from build123d import *

# Parameters (mm, degrees)
SKETCH_1_R           = 2.250000000000002
SKETCH_1_R_2         = 2.2500000000000027
EXTRUDE_1_DEPTH      = 4
EXTRUDE_2_DEPTH      = 58
EXTRUDE_3_REACH      = 110.805
EXTRUDE_3_END_RADIUS = 44.19999999999999
CUT_EXTRUDE_1_REACH  = 89.17
SKETCH_4_R           = 3.0000000000000013
FILLET_1_R           = 2
CHAMFER_1_SIZE       = 2
EXTRUDE_4_DEPTH      = 58
EXTRUDE_5_DEPTH      = 6.412205295
SKETCH_8_R           = 1.5000000000000042
SKETCH_8_R_2         = 1.5000000000000009
SKETCH_8_R_3         = 1.500000000000004
SKETCH_8_R_4         = 1.500000000000017
SKETCH_8_R_5         = 1.5000000000000173
CUT_EXTRUDE_2_DEPTH  = 5
CHAMFER_2_SIZE       = 0.5
CHAMFER_3_SIZE       = 3


with BuildPart() as part:
    # Эскиз1 → Бобышка-Вытянуть1 (new body)
    with BuildSketch(Plane(origin=(0, 0, 0), x_dir=(1, 0, 0), z_dir=(0, 1, 0))):
        with BuildLine():
            Line((-42.93077537059159, -10.516107934012744), (-39.47597367549217, -16.5))
            Line((-39.47597367549216, -16.5), (-34.49999999999999, -16.5))
            Line((-34.49999999999999, -16.5), (-34.49999999999999, -3.5000000000000013))
            Line((-34.49999999999999, -3.5000000000000013), (-34.49999999999999, 3.5000000000000013))
            Line((-34.49999999999999, 3.5000000000000018), (-34.49999999999999, 17.5))
            Line((-34.49999999999999, 17.5), (-25.274990747593094, 17.499999999999996))
            Line((-25.274990747593094, 17.499999999999996), (-16, 26.77499074759315))
            Line((-16, 26.77499074759315), (16, 26.77499074759315))
            Line((16, 26.77499074759315), (25.274990747593094, 17.499999999999996))
            Line((25.274990747593094, 17.499999999999996), (34.50000000000001, 17.5))
            Line((34.50000000000001, 17.5), (34.50000000000001, 3.5000000000000013))
            Line((34.50000000000001, 3.5000000000000013), (34.5, -3.5000000000000013))
            Line((34.5, -3.5000000000000018), (34.5, -16.5))
            Line((34.5, -16.5), (39.475973675492156, -16.5))
            Line((39.475973675492156, -16.5), (42.9307753705916, -10.516107934012684))
            ThreePointArc((42.93077537059159, -10.516107934012682), (44.199999999999974, 1.599e-14), (42.93077537059159, 10.516107934012718))
            Line((42.93077537059159, 10.516107934012716), (30.572604305089854, 31.92108810808932))
            ThreePointArc((30.57260430508986, 31.92108810808933), (22.099999999999994, 38.27832284727222), (12.358171065501741, 42.43719604210199))
            Line((12.358171065501741, 42.437196042101974), (-12.358171065501741, 42.437196042101974))
            ThreePointArc((-12.358171065501743, 42.43719604210198), (-22.099999999999994, 38.278322847272186), (-30.572604305089868, 31.921088108089307))
            Line((-30.572604305089865, 31.9210881080893), (-42.930775370591604, 10.5161079340127))
            ThreePointArc((-42.930775370591604, 10.516107934012702), (-44.19999999999999, -1.954e-14), (-42.93077537059159, -10.516107934012746))
        make_face()
        with Locations(Location((-39, 0, 0), (0, 0, 270))):
            Circle(SKETCH_1_R, mode=Mode.SUBTRACT)
        with Locations(Location((39, 0, 0), (0, 0, 270))):
            Circle(SKETCH_1_R, mode=Mode.SUBTRACT)
        with Locations(Location((-19.50000000000016, 33.77499074759302, 0), (0, 0, 270))):
            Circle(SKETCH_1_R_2, mode=Mode.SUBTRACT)
        with BuildLine():
            Line((-8, 36.024990747593144), (8, 36.024990747593144))
            ThreePointArc((8, 36.024990747593144), (10.25, 33.774990747593144), (7.999999999999998, 31.524990747593144))
            Line((7.999999999999998, 31.524990747593144), (-7.999999999999998, 31.524990747593144))
            ThreePointArc((-7.999999999999998, 31.524990747593144), (-10.25, 33.774990747593144), (-8, 36.024990747593144))
        make_face(mode=Mode.SUBTRACT)
        with Locations(Location((19.499999999999925, 33.77499074759315, 0), (0, 0, 270))):
            Circle(SKETCH_1_R_2, mode=Mode.SUBTRACT)
    extrude(amount=EXTRUDE_1_DEPTH)

    # Эскиз2 → Бобышка-Вытянуть2 (add)
    with BuildSketch(Plane(origin=(0, 4, 0), x_dir=(1, 0, 0), z_dir=(0, 1, 0))):
        with BuildLine():
            ThreePointArc((-42.9307753705916, 10.516107934012743), (-43.16465657781108, 9.51064784962775), (-43.37499279538843, 8.50000000000001))
            Line((-43.37499279538844, 8.50000000000001), (-34.499999999999986, 8.500000000000005))
            Line((-34.499999999999986, 8.500000000000005), (-34.49999999999999, 16.5))
            Line((-34.49999999999999, 16.5), (-39.47597367549217, 16.5))
            Line((-39.47597367549217, 16.5), (-42.9307753705916, 10.516107934012743))
        make_face()
        with BuildLine():
            Line((-34.499999999999986, -8.500000000000005), (-43.37499279538844, -8.50000000000001))
            ThreePointArc((-43.37499279538843, -8.50000000000001), (-43.16465657781108, -9.51064784962775), (-42.9307753705916, -10.516107934012743))
            Line((-42.9307753705916, -10.516107934012743), (-39.47597367549217, -16.5))
            Line((-39.47597367549217, -16.5), (-34.49999999999999, -16.5))
            Line((-34.49999999999999, -16.5), (-34.499999999999986, -8.500000000000005))
        make_face()
        with BuildLine():
            Line((34.499999999999986, 8.500000000000005), (43.37499279538844, 8.50000000000001))
            ThreePointArc((43.37499279538845, 8.50000000000001), (43.16465657781109, 9.510647849627738), (42.930775370591604, 10.51610793401272))
            Line((42.930775370591604, 10.516107934012684), (39.475973675492156, 16.5))
            Line((39.475973675492156, 16.5), (34.5, 16.5))
            Line((34.5, 16.5), (34.499999999999986, 8.500000000000005))
        make_face()
        with BuildLine():
            ThreePointArc((42.93077537059162, -10.516107934012688), (43.164656577811115, -9.510647849627723), (43.37499279538845, -8.50000000000001))
            Line((43.37499279538844, -8.50000000000001), (34.499999999999986, -8.500000000000005))
            Line((34.499999999999986, -8.500000000000005), (34.5, -16.5))
            Line((34.5, -16.5), (39.475973675492156, -16.5))
            Line((39.475973675492156, -16.5), (42.930775370591604, -10.516107934012684))
        make_face()
    extrude(amount=EXTRUDE_2_DEPTH)

    # Бобышка-Вытянуть3: up to this cylinder (the profile starts inside it)
    extrude_3_end = Plane(origin=(0, 61.785199, 0), z_dir=(0, -1, 0)) * Cylinder(EXTRUDE_3_END_RADIUS, 311.01, mode=Mode.PRIVATE)
    # Эскиз3 → Бобышка-Вытянуть3 (add, up to the surface)
    with BuildSketch(Plane(origin=(-34.49999999999999, 0, 0), x_dir=(0, 0, -1), z_dir=(1, 0, 0)), mode=Mode.PRIVATE) as extrude_3_sk1:
        Polygon((-8.500000000000007, 62.00000000000001), (8.500000000000005, 62.00000000000001), (8.500000000000005, 48.87009446294909), (0, 59.00000000000001), (-8.500000000000005, 48.87009446294909), align=None)
    extrude_3_tool1 = extrude(extrude_3_sk1.sketch, amount=-EXTRUDE_3_REACH, mode=Mode.PRIVATE) & extrude_3_end
    extrude_3 = extrude_3_tool1.solids().sort_by_distance((-34.5, 61.785199, 0))[0]
    add(extrude_3)

    # Зеркальное отражение1: Бобышка-Вытянуть3 across plane
    add(extrude_3.mirror(Plane(origin=(0, 0, 0), x_dir=(0, 0, 1), z_dir=(1, 0, 0))))

    # Вырез-Вытянуть1: up to this face of the body (flat: up to its plane)
    cut_extrude_1_end = Plane(part.part.faces().sort_by_distance((44.00427315, 4, 0))[0])
    # Эскиз4 → Вырез-Вытянуть1 (cut, up to the picked face)
    with BuildSketch(Plane(origin=(0, 62.00000000000001, 0), x_dir=(1, 0, 0), z_dir=(0, 1, 0)), mode=Mode.PRIVATE) as cut_extrude_1_sk1:
        with Locations(Location((-39, 0, 0), (0, 0, 270))):
            Circle(SKETCH_4_R)
    cut_extrude_1_tool1 = split(extrude(cut_extrude_1_sk1.sketch, amount=-CUT_EXTRUDE_1_REACH, mode=Mode.PRIVATE), bisect_by=cut_extrude_1_end, keep=Keep.BOTH, mode=Mode.PRIVATE)
    # Эскиз4 → Вырез-Вытянуть1 (cut, up to the picked face)
    with BuildSketch(Plane(origin=(0, 62.00000000000001, 0), x_dir=(1, 0, 0), z_dir=(0, 1, 0)), mode=Mode.PRIVATE) as cut_extrude_1_sk2:
        with Locations(Location((39, 0, 0), (0, 0, 270))):
            Circle(SKETCH_4_R)
    cut_extrude_1_tool2 = split(extrude(cut_extrude_1_sk2.sketch, amount=-CUT_EXTRUDE_1_REACH, mode=Mode.PRIVATE), bisect_by=cut_extrude_1_end, keep=Keep.BOTH, mode=Mode.PRIVATE)
    add(cut_extrude_1_tool1.solids().sort_by(Axis((-39, 62, 0), (0, -1, 0)))[0], mode=Mode.SUBTRACT)
    add(cut_extrude_1_tool2.solids().sort_by(Axis((39, 62, 0), (0, -1, 0)))[0], mode=Mode.SUBTRACT)

    # Скругление1
    fillet_1_edges = [part.edges().sort_by_distance(p)[0] for p in [
        (35.249999999999986, 59.00000000000001, 0),
        (43.1, 59.00000000000001, 0),
        (-43.1, 59.00000000000001, 0),
        (-35.249999999999986, 59.00000000000001, 0),
    ]]
    fillet(fillet_1_edges, radius=FILLET_1_R)

    # Фаска1
    chamfer_1_edges = [part.edges().sort_by_distance(p)[0] for p in [
        (-19.50000000000016, 4, -36.02499074759302),
        (19.499999999999925, 4, -36.02499074759315),
        (39, 4, -2.250000000000002),
        (-39, 4, -2.250000000000002),
    ]]
    chamfer(chamfer_1_edges, length=CHAMFER_1_SIZE)

    # Эскиз6 → Бобышка-Вытянуть4 (add)
    with BuildSketch(Plane(origin=(0, 4, 0), x_dir=(1, 0, 0), z_dir=(0, 1, 0))):
        with BuildLine():
            Line((8, 36.024990747593144), (5.000000000000001, 36.024990747593144))
            Line((5.000000000000001, 36.024990747593144), (5, 42.437196042101974))
            Line((5, 42.437196042101974), (12.358171065501741, 42.437196042101974))
            ThreePointArc((12.358171065501741, 42.437196042101974), (14.696759256079767, 41.68507247647332), (16.989949980131733, 40.8041860557544))
            Line((16.989949980131733, 40.8041860557544), (15, 36.02499074759314))
            Line((15, 36.02499074759314), (8, 36.024990747593144))
        make_face()
        with BuildLine():
            Line((-12.358171065501741, 42.437196042101974), (-5, 42.437196042101974))
            Line((-5, 42.437196042101974), (-5.000000000000001, 36.024990747593144))
            Line((-5.000000000000001, 36.024990747593144), (-8, 36.024990747593144))
            Line((-8, 36.024990747593144), (-15, 36.02499074759314))
            Line((-15, 36.02499074759314), (-16.989949980131733, 40.8041860557544))
            ThreePointArc((-16.989949980131733, 40.8041860557544), (-14.696759256079767, 41.685072476473316), (-12.358171065501741, 42.437196042101974))
        make_face()
    extrude(amount=EXTRUDE_4_DEPTH)

    # Эскиз7 → Бобышка-Вытянуть5 (add)
    with BuildSketch(Plane.XY.offset(-36.024990747593144)):
        Polygon((-5.000000000000001, 62.00000000000001), (-5, 53.04123203702888), (0, 59.00000000000001), (5.000000000000003, 53.04123203702888), (5.000000000000001, 62.00000000000001), align=None)
    extrude(amount=-EXTRUDE_5_DEPTH)

    # Эскиз8 → Вырез-Вытянуть2 (cut)
    with BuildSketch(Plane(origin=(0, 62.00000000000001, 0), x_dir=(1, 0, 0), z_dir=(0, 1, 0))):
        with Locations(Location((38.99999999999992, 8, 0), (0, 0, 270))):
            Circle(SKETCH_8_R)
        with Locations(Location((8, 39.23109339484765, 0), (0, 0, 270))):
            Circle(SKETCH_8_R_2)
        with Locations(Location((38.99999999999992, -8, 0), (0, 0, 90))):
            Circle(SKETCH_8_R_3)
        with Locations(Location((-8, 39.23109339484765, 0), (0, 0, 90))):
            Circle(SKETCH_8_R)
        with Locations(Location((-38.999999999999865, -8.000000000000222, 0), (0, 0, 270))):
            Circle(SKETCH_8_R_4)
        with Locations(Location((-38.99999999999998, 7.999999999999556, 0), (0, 0, 90))):
            Circle(SKETCH_8_R_5)
    extrude(amount=-CUT_EXTRUDE_2_DEPTH, mode=Mode.SUBTRACT)

    # Фаска2
    chamfer_2_edges = [part.edges().sort_by_distance(p)[0] for p in [
        (8, 62.00000000000001, -40.73109339484765),
        (40.22474487139151, 62.00000000000001, 7.133974596215554),
        (-8, 62.00000000000001, -37.73109339484764),
        (-39.8660254037844, 62.00000000000001, 9.224744871391763),
        (-38.13397459621573, 62.00000000000001, -9.224744871391302),
        (37.775255128608336, 62.00000000000001, -7.133974596215554),
    ]]
    chamfer(chamfer_2_edges, length=CHAMFER_2_SIZE)

    # Фаска3
    chamfer_3_edges = [part.edges().sort_by_distance(p)[0] for p in [
        (-38.93749639769421, 4, 8.500000000000007),
        (38.93749639769421, 4, -8.500000000000007),
        (38.93749639769421, 4, 8.500000000000009),
        (5, 4, -39.23109339484756),
        (-5, 4, -39.23109339484756),
        (-38.93749639769421, 4, -8.500000000000009),
    ]]
    chamfer(chamfer_3_edges, length=CHAMFER_3_SIZE)


solid = part.part
Design review of the part built by this model. Coordinates are the model's own, in mm. A direction names the side the tool comes from. Coordinates: 2 decimals unless noted, no trailing zeros. Order: outer loops, then holes, each group sorted by start corner. A loop starts at its lowest first (then second) coordinate and runs counter-clockwise, first axis right, second up. Notation, with made-up numbers: M 77,28.5 L 121,28.5 A28 cw 121,59.5 Z; hole C 28,-27.75 d6. An arc over 180 degrees is marked long. Use a Markdown table: item, result.
(1) For P1, Ø1.2, axis at x = -31.5, y = 2, coming from the +Z side; P2, Ø5, axis at y = 30, z = -38.5, coming from the +X side; P3, Ø7, axis at x = -38.5, y = 32.5, coming from the -Z side, all flat-tipped, find the tip position at first contact; note any pin that passes through.
Worked answers:
| item | result |
|---|---|
| P1 | stops at z = -17.5 |
| P2 | stops at x = 16.99 |
| P3 | stops at z = -16.5 |
(2) Draft analysis for pull direction Y (two halves, no side actions). For faces 6 (the cylindrical face through (-35.26, 57.89, -0.02)), 7 (the flat face through (39, 57, 8)), 8 (the flat face through (39.584, 23.677, -16.312)), state which applies: released by +Y, released by -Y, zero draft, split by the parting line, or undercut.
Worked answers:
| item | result |
|---|---|
| face 6 | undercut |
| face 7 | released by +Y |
| face 8 | zero draft |
(3) Wall thickness on probe 1 along X at (y, z) = (60.25, 0); probe 2 along X at (y, z) = (0.7, 0); probe 3 along Z at (x, y) = (-39, 22): over which ranges is each line inside the solid? List them lowest first.
Worked answers:
| item | result |
|---|---|
| probe 1 | x = -44.2 to -42, -36 to -34.5, 34.5 to 36, 42 to 44.2 |
| probe 2 | x = -44.2 to -41.25, -36.75 to -34.5, 34.5 to 36.75, 41.25 to 44.2 |
| probe 3 | z = -16.5 to -8.5, 8.5 to 16.5 |
(4) Add section C-C (z = -23). Give the boundary of the cut face in (x, y) (3 decimals), then the cut area to 3 significant figures.
Worked answers:
| item | result |
|---|---|
| outline | M -35.723,0 L -19.775,0 L -19.775,4 L -35.723,4 Z; M 19.775,0 L 35.723,0 L 35.723,4 L 19.775,4 Z |
| area | 128 mm2 |
(5) For faces 1 (the flat face through (34.5, 31, -12)), 2 (the flat face through (-39, 57, 8)), 3 (the flat face through (39.269, 52.964, -5.065)), 4 (the cylindrical face through (-17.27, 0.99, -34.07)), 5 (the flat face through (-2.535, 55.979, -39.186)), list the 3-axis set-ups (+Z, -Z, +X, -X, +Y, -Y) from which the entire face can be reached by the end or side of a thin tool; tool diameter is ignored.
Worked answers:
| item | result |
|---|---|
| face 1 | +Z, +Y, -Y |
| face 2 | +Y |
| face 3 | +X, -X |
| face 4 | +Y, -Y |
| face 5 | +Z, -Z |
(6) Add section A-A (y = 26). Count the separate pieces of the cut face and the enclosed holes in it, then the cut area to 3 significant figures.
Worked answers:
| item | result |
|---|---|
| separate pieces | 6 |
| enclosed holes | 0 |
| area | 367 mm2 |
(7) Add section B-B (x = -19.5). Give the boundary of the cut face in (y, z) (3 decimals).
Worked answers:
| item | result |
|---|---|
| outline | M 0,-39.666 L 4,-39.666 L 4,-38.025 L 2,-36.025 L 0,-36.025 Z; M 0,-31.525 L 2,-31.525 L 4,-29.525 L 4,-23.275 L 0,-23.275 Z |
